Check sheet for the modelled part. Datum: model origin and axes. Units: mm. A direction names the side the tool comes from. Round coordinates to 2 decimals unless told otherwise and drop trailing zeros. Order: outer loops, then holes, each group sorted by start corner. A loop starts at its lowest first (then second) coordinate and runs counter-clockwise, first axis right, second up. Notation, with made-up numbers: (81, 79.25) -> (134, 79.25) arc R36 ccw to (134, 118.25) -> close; hole circle Ø1 at (74.25, 49.5). An arc over 180 degrees is marked (long way). Answer in a Markdown table with one row per item.
Autodesk Fusion 360 part; units mm, degrees
sketch "Sketch1" plane through (0, 0, 0) normal (0, 0, 1) x (1, 0, 0)
  line L0 (-50, 18.3) -> (-50, -10.5)
  line L1 (-50, -10.5) -> (-32.4, -10.5)
  line L2 (-32.4, -10.5) -> (-32.4, -13.8)
  line L3 (-32.4, -13.8) -> (-7.6, -13.8)
  line L4 (-7.6, -13.8) -> (-7.6, -10.5)
  line L5 (-7.6, -10.5) -> (10, -10.5)
  line L6 (10, -10.5) -> (10, 18.3)
  line L7 (10, 18.3) -> (-7.6, 18.3)
  line L8 (-7.6, 18.3) -> (-7.6, 21.6)
  line L9 (-7.6, 21.6) -> (-32.4, 21.6)
  line L10 (-32.4, 21.6) -> (-32.4, 18.3)
  line L11 (-32.4, 18.3) -> (-50, 18.3)
  line L12 (-47, 15.4) -> (7, 15.4)
  line L13 (7, 15.4) -> (7, -7.6)
  line L14 (7, -7.6) -> (-47, -7.6)
  line L15 (-47, -7.6) -> (-47, 15.4)
  line L16 (-50, 3.9) -> (-47, 3.9)
  line L17 (-20, 15.4) -> (-20, 21.6)
  line L18 (-40, 15.4) -> (-40, 7.4)
  line L19 (-40, 7.4) -> (-32, 7.4)
  line L20 (-32, 7.4) -> (-32, 15.4)
  line L21 (-45, -6.6) -> (5, -6.6)
  line L22 (5, -6.6) -> (5, -4.1)
  line L23 (5, -4.1) -> (-45, -4.1)
  line L24 (-45, -4.1) -> (-45, -6.6)
  line L25 (-20, -6.6) -> (-20, -7.6)
  line L26 (-45, 14.4) -> (5, 14.4)
  line L27 (5, 14.4) -> (5, 11.9)
  line L28 (-45, 11.9) -> (-45, 14.4)
  line L29 (5, 11.9) -> (-45, 11.9)
  line L30 (-45, 11.9) -> (-45, -4.1)
  line L31 (5, 11.9) -> (5, -4.1)
  line L32 (-31, 15.4) -> (-31, 16.9)
  line L33 (-31, 16.9) -> (-48.5, 16.9)
  line L34 (-48.5, 16.9) -> (-48.5, -4.5956)
  line L35 (-48.5, -4.5956) -> (-47, -4.5956)
  line L36 (-41, 15.4) -> (-41, 16.9)
  dimension "d1" = 60
  dimension "d2" = 24.8
  dimension "d3" = 28.8
  dimension "d4" = 35.4
  dimension "d8" = 23
  dimension "d9" = 54
  dimension "d10" = 8
  dimension "d11" = 8
  dimension "d12" = 7
  dimension "d13" = 1
  dimension "d14" = 2.5
  dimension "d15" = 50
  dimension "d153" = 1.5
  dimension "d154" = 1.5
  dimension "d155" = 1
  dimension "d156" = 1
extrude "Extrude2" add sketch "Sketch1" along normal blind 18 contours L12 L32 L33 L36 | L12 L18 L20 L26 | L18 L20 L26 L29 | L18 L19 L20 L29
extrude "Extrude3" add sketch "Sketch1" along normal blind 14 contours L12 L15 L16 L33 L34 L36 | L12 L14 L15 L18 L21 L24 L25 L26 L28 L30 | L12 L13 L14 L20 L21 L22 L25 L26 L27 L31 | L21 L22 L23 L24 | L18 L26 L28 L29 | L20 L26 L27 L29 | L18 L19 L20 L23 L29 L30 L31
extrude "Extrude5" add sketch "Sketch1" along normal blind 2 contours L0 L9 L10 L11 L12 L16 L17 L32 L33 L34 | L0 L1 L2 L3 L4 L5 L6 L7 L8 L9 L12 L13 L14 L15 L16 L17 L34 L35 | L12 L15 L16 L33 L34 L36 | L15 L16 L34 L35 | L12 L14 L15 L18 L21 L24 L25 L26 L28 L30 | L12 L32 L33 L36 | L12 L13 L14 L20 L21 L22 L25 L26 L27 L31 | L12 L18 L20 L26 | L18 L19 L20 L29 | L18 L19 L20 L23 L29 L30 L31
chamfer "Chamfer5" distance 1 angle 45 2 edges at (-40, 15.4, 16) (-32, 15.4, 16)
fillet "Fillet2" radius 2 12 edges at (-7.6, 18.3, 1) (-7.6, 21.6, 1) (-32.4, 21.6, 1) (-32.4, 18.3, 1) (-50, 18.3, 1) (-50, -10.5, 1) (-32.4, -10.5, 1) (-32.4, -13.8, 1) (-7.6, -10.5, 1) (-7.6, -13.8, 1) (10, -10.5, 1) (10, 18.3, 1)
fillet "Fillet26" radius 2 4 edges at (7, 15.4, 8) (7, -7.6, 8) (-47, -7.6, 8) (-48.5, 16.9, 8)
Item 1: Depth check by flat-ended pin: P1, Ø3, axis at y = 12.5, z = 16, coming from the +X side; P2, Ø2, axis at x = -1, z = 0.5, coming from the -Y side; P3, Ø2, axis at x = -35, z = 16.5, coming from the -Y side. Enter the tip coordinate at first touch or a pass-through.
Result sheet:
| item | result |
|---|---|
| P1 | stops at x = -32 |
| P2 | stops at y = -10.5 |
| P3 | stops at y = 7.4 |
Item 2: Cross-section at B-B (x = 1.5). Record the boundary of the cut face in (y, z).
Result sheet:
| item | result |
|---|---|
| outline | (-10.5, 0) -> (18.3, 0) -> (18.3, 2) -> (15.4, 2) -> (15.4, 14) -> (-7.6, 14) -> (-7.6, 2) -> (-10.5, 2) -> close |
Item 3: Cross-section at C-C (z = 13.25). Record the boundary of the cut face in (x, y), and give its area (3 significant figures).
Result sheet:
| item | result |
|---|---|
| outline | (-48.5, 3.9) -> (-47, 3.9) -> (-47, -5.6) arc R2 ccw to (-45, -7.6) -> (5, -7.6) arc R2 ccw to (7, -5.6) -> (7, 13.4) arc R2 ccw to (5, 15.4) -> (-31, 15.4) -> (-31, 16.9) -> (-46.5, 16.9) arc R2 ccw to (-48.5, 14.9) -> close |
| area | 1,280 mm^2 |
Item 4: Set-up check for faces 1 (the flat face through (-41, 18.3, 1)), 2 (the flat face through (1, -10.5, 1)), 3 (the flat face through (7, 4, 8)), 4 (the flat face through (-32, 11, 16)): record each of +Z, -Z, +X, -X, +Y, -Y from which the full face is reachable in a straight line by a thin tool's end or side.
Result sheet:
| item | result |
|---|---|
| face 1 | +Z, -Z, -X, +Y |
| face 2 | +Z, -Z, +X, -Y |
| face 3 | +Z, +X, +Y, -Y |
| face 4 | +Z, +X, -Y |
Item 5: Cross-section at A-A (y = 10). Record the boundary of the cut face in (x, z).
Result sheet:
| item | result |
|---|---|
| outline | (-50, 0) -> (10, 0) -> (10, 2) -> (7, 2) -> (7, 14) -> (-32, 14) -> (-32, 18) -> (-40, 18) -> (-40, 14) -> (-48.5, 14) -> (-48.5, 2) -> (-50, 2) -> close |
Item 6: Cross-section at D-D (y = 5). Record the boundary of the cut face in (x, z), and give its area (3 significant figures).
Result sheet:
| item | result |
|---|---|
| outline | (-50, 0) -> (10, 0) -> (10, 2) -> (7, 2) -> (7, 14) -> (-48.5, 14) -> (-48.5, 2) -> (-50, 2) -> close |
| area | 786 mm^2 |
Item 7: Scan lines: line 1 (Z direction, x = -4.5, y = 11); line 2 (Z direction, x = -45, y = -8); line 3 (X direction, y = -2, z = 8.25). Record each from-to range of solid material in increasing order. Write a range as [from, to].
Result sheet:
| item | result |
|---|---|
| line 1 | z = [0, 14] |
| line 2 | z = [0, 2] |
| line 3 | x = [-47, 7] |
